Source: CAD feature listing. Evaluate the final solid. Frame: model axes, mm. Face numbers are marked on the shaded views. Give positions to 0.01 mm unless a question says otherwise; leave off trailing zeros. Order: outer loops, then holes, each group sorted by start corner. A loop starts at its lowest first (then second) coordinate and runs counter-clockwise, first axis right, second up. Notation, with made-up numbers: M -31,63 L 3,63 A29 cw 3,97 Z; hole C 10,-7 d8. An arc over 180 degrees is marked long. Use CSV: the item, a comma, the result in double quotes. Start each with the question number.
Item 1: Ray query, probe 1 along Z at (x, y) = (1.2, -1.25); probe 2 along Z at (x, y) = (-0.5, -0.7); probe 3 along Y at (x, z) = (-1.3, -1). Return the intervals inside material, ascending. Write a range as from..to.
Item 2: First-contact query: pin 1 (1 mm diameter, centred on y = 1, z = -10, fed in from +X); pin 2 (2 mm diameter, centred on x = -0.5, y = 1.5, fed in from -Z); pin 3 (1 mm diameter, centred on x = 1.5, y = 1.5, fed in from -Z); pin 4 (1.5 mm diameter, centred on x = 1.5, z = -1, fed in from -Y). Flat tips, straight axial feed; report the tip coordinate or a pass-through.
Item 3: Pull-direction query (Y, two-part tool) for the marked faces 1, 2 and 3; classes: +Y half, -Y half, draft (parallel to the pull), parting line (faces both ways), or undercut.
Item 4: Section query B-B on x = 0.35. Return loops of the section in (y, z).
Item 5: Section query D-D on y = 1.85. Return loops of the section in (x, z), and give its area (3 significant figures).
Item 6: Section query A-A on y = 0. Return loops of the section in (x, z), and give its area (3 significant figures).
Item 7: Section query C-C on z = -3.25. Return loops of the section in (x, y), and give its area (3 significant figures).
from build123d import *

# Parameters (mm, degrees)
SKETCH_1_W          = 2.208
SKETCH_1_H          = 2.028
SKETCH_2_R          = 1.5
EXTRUDE_1_DEPTH     = 12
CUT_EXTRUDE_1_DEPTH = 1.872


with BuildPart() as part:
    # 草图1 → 旋转1 (revolve)
    with BuildSketch(Plane.XZ, mode=Mode.PRIVATE) as revolve_1_sk:
        with Locations((1.104, 1.014)):
            Rectangle(SKETCH_1_W, SKETCH_1_H)
    revolve(revolve_1_sk.sketch.rotate(Axis((0, 0, 2.028), (0, 0, -1)), 270), axis=Axis((0, 0, 2.028), (0, 0, -1)))

    # 草图2 → 凸台-拉伸1 (add)
    with BuildSketch(Plane(origin=(0, 0, 0), x_dir=(-1, 0, 0), z_dir=(0, 0, -1))):
        with Locations(Location((0, 0, 0), (0, 0, 90))):
            Circle(SKETCH_2_R)
    extrude(amount=EXTRUDE_1_DEPTH)

    # 草图3 → 切除-拉伸1 (cut)
    with BuildSketch(Plane.XY.offset(2.028)):
        Polygon((0.9936, -0.573655227), (0.9936, 0.573655227), (0, 1.147310455), (-0.9936, 0.573655227), (-0.9936, -0.573655227), (0, -1.147310455), align=None)
    extrude(amount=-CUT_EXTRUDE_1_DEPTH, mode=Mode.SUBTRACT)


solid = part.part
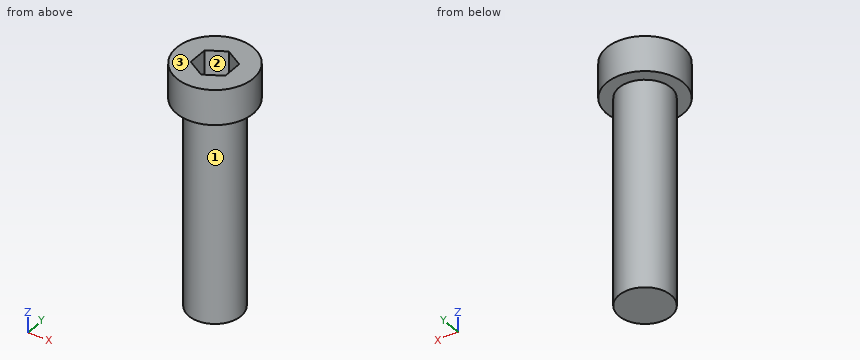
Verdict:
1,probe 1,"0..2.03"
1,probe 2,"-12..0.16"
1,probe 3,"-0.75..0.75"
2,pin 1,"x = 1.41"
2,pin 2,"z = -12"
2,pin 3,"z = 0"
2,pin 4,"y = -1.3"
3,face 1,"parting line"
3,face 2,"undercut"
3,face 3,"draft"
4,outline,"M -2.18,0 L -1.46,0 L -1.46,-12 L 1.46,-12 L 1.46,0 L 2.18,0 L 2.18,2.03 L 0.95,2.03 L 0.95,0.16 L -0.95,0.16 L -0.95,2.03 L -2.18,2.03 Z"
5,outline,"M -1.21,0 L 1.21,0 L 1.21,2.03 L -1.21,2.03 Z"
5,area,"4.89 mm2"
6,outline,"M -2.21,0 L -1.5,0 L -1.5,-12 L 1.5,-12 L 1.5,0 L 2.21,0 L 2.21,2.03 L 0.99,2.03 L 0.99,0.16 L -0.99,0.16 L -0.99,2.03 L -2.21,2.03 Z"
6,area,"41.2 mm2"
7,outline,"C 0,0 d3"
7,area,"7.07 mm2"
